Could you check a few things on this model? Use its own coordinates, in mm. A direction names the side the tool comes from. Give positions to 0.01 mm unless a question says otherwise; leave off trailing zeros. Loops run counter-clockwise (first coordinate to the right, second up) from the corner with the lowest first, then second, coordinate; pieces in that order, holes last. Notation, with made-up numbers: M 82.25,-13 L 132.25,-13 A27 ccw 132.25,18 Z; hole C 48,-32 d5. An arc over 180 degrees is marked long. Answer in a Markdown table with one row per item. Add a question column.
1. Which directions (+Z, -Z, +X, -X, +Y, -Y) give clear straight access to the entire face, cutting with the end or side of a thin tool? Please do faces 1 (the cylindrical face through (34.021, 1.972, -166.445)), 2 (the cylindrical face through (16.539, 1.972, -184.316)).
2. Thinking about a two-plate mould opening in Z: for faces 3 (the cylindrical face through (15.684, 1.972, -16.539)), 4 (the flat face through (240, 4, -101)), 5 (the cylindrical face through (33.555, 1.972, -34.021)), which applies, released by +Z, released by -Z, zero draft, split by the parting line, or undercut?
3. If we section it at D-D on y = 1.55: List the corners of the cut face in (x, z) for me, then the cut area to 3 significant figures.
4. If we section it at B-B on x = 119.5: List the corners of the cut face in (y, z) for me.
5. I need wall thicknesses on line 1 along Z through (x, y) = (250.5, 2.4); line 2 along X through (y, z) = (3.6, -58.5); line 3 along Z through (x, y) = (208.5, 0.3). Which ranges of each line are inside material? Lowest first, please. Write a range as from..to.
6. If we section it at C-C on z = -80.5: List the corners of the cut face in (x, y) for me.
7. If we section it at A-A on x = 229: List the corners of the cut face in (y, z) for me, then the cut area to 3 significant figures.
8. I'm going to push flat-ended pins straight in: pin 1 Ø1.2 at (y, z) = (1.5, -118.5) entering from +X; pin 2 Ø10 at (x, z) = (277.5, -45.5) entering from -Y. Where does each tip first touch, or does it pass through?
```python
from build123d import *

# Parameters (mm, degrees)
BOSS_EXTRUDE1_DEPTH = 4


with BuildPart() as part:
    # Sketch1 → Boss-Extrude1 (new body)
    with BuildSketch(Plane(origin=(0, 0, 0), x_dir=(1, 0, 0), z_dir=(0, 1, 0))):
        with BuildLine():
            Line((55, 0), (280, 0))
            ThreePointArc((280, 0), (318.890872965, 16.109127035), (335, 55))
            Line((335, 55), (335, 71))
            Line((335, 71), (248, 71))
            Line((248, 71), (248, 129))
            Line((248, 129), (335, 129))
            Line((335, 129), (335, 145))
            ThreePointArc((335, 145), (318.890872965, 183.890872965), (280, 200))
            Line((280, 200), (55, 200))
            ThreePointArc((55, 200), (16.109127035, 183.890872965), (0, 145))
            Line((0, 145), (0, 55))
            ThreePointArc((0, 55), (16.109127035, 16.109127035), (55, 0))
        make_face()
        with BuildLine():
            Line((55, 25), (280, 25))
            ThreePointArc((280, 25), (297.748239349, 30.813226755), (308.618176043, 46))
            Line((308.618176043, 46), (223, 46))
            Line((223, 46), (223, 154))
            Line((223, 154), (308.618176043, 154))
            ThreePointArc((308.618176043, 154), (297.748239349, 169.186773245), (280, 175))
            Line((280, 175), (55, 175))
            ThreePointArc((55, 175), (33.786796564, 166.213203436), (25, 145))
            Line((25, 145), (25, 55))
            ThreePointArc((25, 55), (33.786796564, 33.786796564), (55, 25))
        make_face(mode=Mode.SUBTRACT)
    extrude(amount=BOSS_EXTRUDE1_DEPTH)


solid = part.part
```
Results:
| question | item | result |
|---|---|---|
| 1 | face 1 | +Y, -Y |
| 1 | face 2 | -Z, -X, +Y, -Y |
| 2 | face 3 | released by +Z |
| 2 | face 4 | zero draft |
| 2 | face 5 | undercut |
| 3 | outline | M 0,-145 A55 ccw 55,-200 L 280,-200 A55 ccw 335,-145 L 335,-129 L 248,-129 L 248,-71 L 335,-71 L 335,-55 A55 ccw 280,0 L 55,0 A55 ccw 0,-55 Z; hole M 25,-145 A30 ccw 55,-175 L 280,-175 A30 ccw 308.62,-154 L 223,-154 L 223,-46 L 308.62,-46 A30 ccw 280,-25 L 55,-25 A30 ccw 25,-55 Z |
| 3 | area | 26,800 mm2 |
| 4 | outline | M 0,-200 L 4,-200 L 4,-175 L 0,-175 Z; M 0,-25 L 4,-25 L 4,0 L 0,0 Z |
| 5 | line 1 | -200..-175, -154..-129, -71..-46, -25..0 |
| 5 | line 2 | 0..25, 223..335 |
| 5 | line 3 | -200..-175, -25..0 |
| 6 | outline | M 0,0 L 25,0 L 25,4 L 0,4 Z; M 223,0 L 248,0 L 248,4 L 223,4 Z |
| 7 | outline | M 0,-200 L 4,-200 L 4,-175 L 0,-175 Z; M 0,-154 L 4,-154 L 4,-46 L 0,-46 Z; M 0,-25 L 4,-25 L 4,0 L 0,0 Z |
| 7 | area | 632 mm2 |
| 8 | pin 1 | x = 248 |
| 8 | pin 2 | y = 0 |
